Verification items for this drawing (mm, ordinates from the low corner). A direction names the side the tool comes from. Round coordinates to 2 decimals unless told otherwise and drop trailing zeros. Order: outer loops, then holes, each group sorted by start corner. A loop starts at its lowest first (then second) coordinate and runs counter-clockwise, first axis right, second up. Notation, with made-up numbers: (6, -18) - (24, -18) arc R28 cw to (24, 0) - close; hole circle Ø5 at (26, 89.25). An arc over 180 degrees is marked (long way). Use a Markdown table: item, result. Add a question column.
(1) Access from +Z, -Z, +X, -X, +Y, -Y to the whole of each face (thin tool, end or side, straight path). Record for the marked faces 1 and 2.
(2) Section check C-C on x = 101.5. Record the boundary of the cut face in (y, z).
(3) Mould release check, pull along Y, two halves, no side actions. Record for the marked faces 3, 4 and 5: released by +Y, released by -Y, zero draft, split by the parting line, or undercut.
(4) Thickness scan on line 1 along Y through (x, z) = (102.5, 16); line 2 along X through (y, z) = (104.5, 29.5); line 3 along Y through (x, z) = (159, 42.5). Record the ranges inside material, lowest first. Write a range as [from, to].
(5) Section check D-D on x = 186. Record the boundary of the cut face in (y, z).
(6) Section check B-B on z = 11.5. Record the boundary of the cut face in (x, y).
(7) Section check A-A on y = 121. Record the boundary of the cut face in (x, z), then the cut area to 3 significant figures.
(8) Gauge pin test, flat end, axial feed: P1, Ø4, axis at x = 30.5, y = 96.5, coming from the +Z side. Record the tip position at first contact, or that the pin passes through.
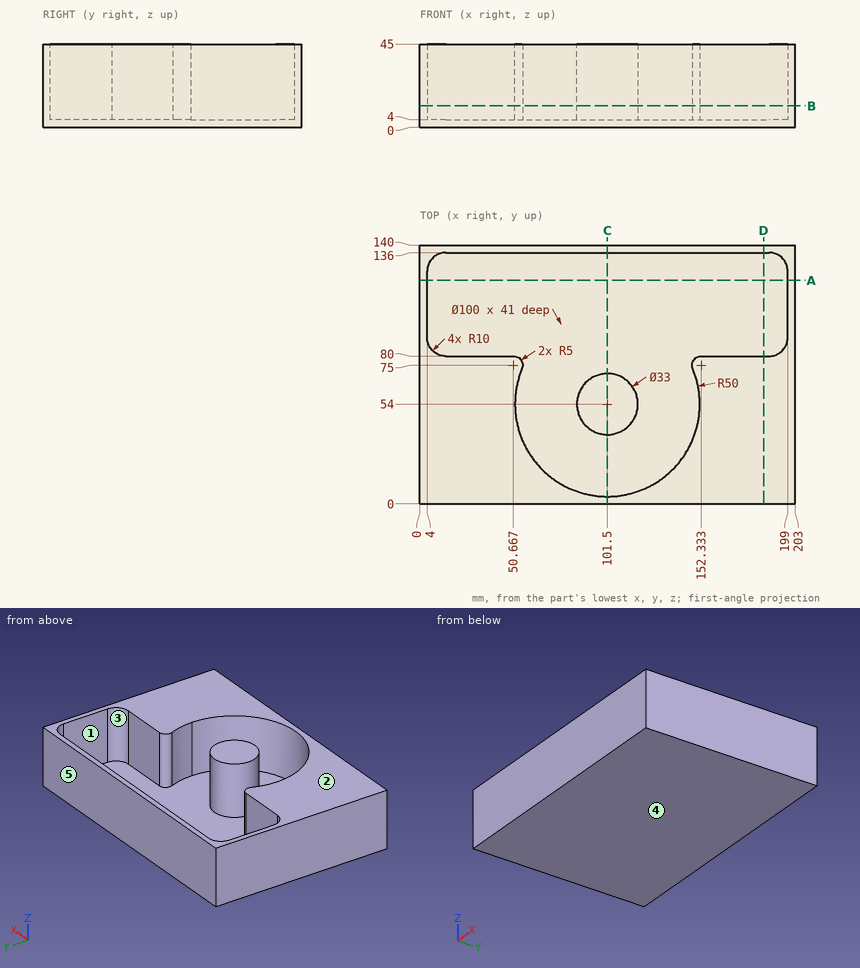
Check sheet entries:
| question | item | result |
|---|---|---|
| 1 | face 1 | +Z |
| 1 | face 2 | +Z, +X, -X, +Y, -Y |
| 2 | outline | (0, 0) - (140, 0) - (140, 45) - (136, 45) - (136, 4) - (70.5, 4) - (70.5, 45) - (37.5, 45) - (37.5, 4) - (4, 4) - (4, 45) - (0, 45) - close |
| 3 | face 3 | undercut |
| 3 | face 4 | zero draft |
| 3 | face 5 | released by +Y |
| 4 | line 1 | y = [0, 4.01], [37.53, 70.47], [136, 140] |
| 4 | line 2 | x = [0, 4], [199, 203] |
| 4 | line 3 | y = [0, 80], [136, 140] |
| 5 | outline | (0, 0) - (140, 0) - (140, 45) - (136, 45) - (136, 4) - (80, 4) - (80, 45) - (0, 45) - close |
| 6 | outline | (0, 0) - (203, 0) - (203, 140) - (0, 140) - close; circle Ø33 at (101.5, 54); hole (4, 90) arc R10 ccw to (14, 80) - (50.67, 80) arc R5 cw to (55.29, 73.09) arc R50 ccw (long way) to (147.71, 73.09) arc R5 cw to (152.33, 80) - (189, 80) arc R10 ccw to (199, 90) - (199, 126) arc R10 ccw to (189, 136) - (14, 136) arc R10 ccw to (4, 126) - close |
| 7 | outline | (0, 0) - (203, 0) - (203, 45) - (199, 45) - (199, 4) - (4, 4) - (4, 45) - (0, 45) - close |
| 7 | area | 1,140 mm2 |
| 8 | P1 | stops at z = 4 |
